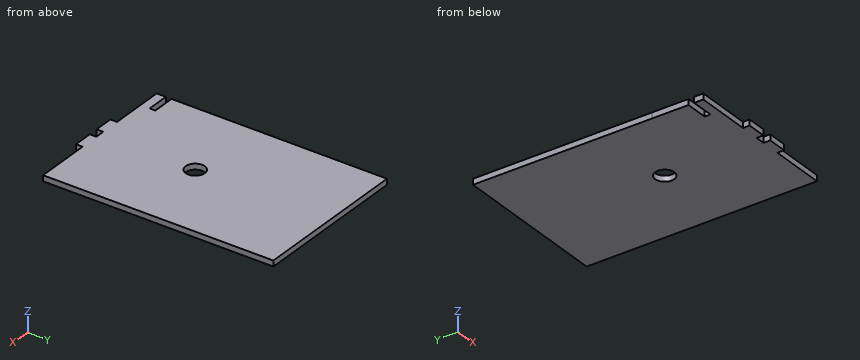
```python
from build123d import *

# Parameters (mm, degrees)
MODEL_R                 = 5
SALIENTE_EXTRUIR1_DEPTH = 3


with BuildPart() as part:
    # Model → Saliente-Extruir1 (new body)
    with BuildSketch(Plane.XY):
        Polygon((43.835480064, -35.842547763), (43.835480064, -32.349014415), (14.885477826, -32.340639111), (14.885479202, -27.550194175), (26.685480393, -27.550194175), (26.685480393, -24.550194175), (14.885480064, -24.550193732), (14.885483847, -5.553308235), (14.885503897, 88.349821578), (97.885505249, 88.349799035), (97.885505249, -32.347086905), (68.935480064, -32.349014415), (68.935480064, -35.842547763), (58.885480064, -35.842547763), (58.885480064, -32.342547763), (53.885480064, -32.342547763), (53.885480064, -35.842547763), align=None)
        with Locations((56.385505249, 17.649799035)):
            Circle(MODEL_R, mode=Mode.SUBTRACT)
    extrude(amount=SALIENTE_EXTRUIR1_DEPTH)


solid = part.part
```
The listing builds one solid part. Answer for the finished solid, in the listing's coordinates (mm). Give positions to 0.01 mm unless a question says otherwise; leave off trailing zeros. Order: outer loops, then holes, each group sorted by start corner. A loop starts at its lowest first (then second) coordinate and runs counter-clockwise, first axis right, second up. Notation, with made-up numbers: (-4.75, 36.25) - (9.25, 36.25) arc R19 cw to (9.25, 50.25) - close; hole circle Ø8 at (8.5, -26.5). An arc over 180 degrees is marked (long way). Use one line per item in the form item = value. Start each with the question number.
(1) A cutting plane is placed at A-A, the plane x = 57. Write down the section's boundary in (y, z).
(2) A cutting plane is placed at B-B, the plane z = 1.45. Write down the section's boundary in (x, y).
(3) Consider line 1 (Y direction, x = 91, z = 2.6); line 2 (X direction, y = -27, z = 2.3); line 3 (Y direction, x = 55, z = 1.3). Determine where each line is inside the solid, lowest interval first. Write a range as from..to.
(4) A cutting plane is placed at D-D, the plane x = 42. Write down the section's boundary in (y, z).
(5) A cutting plane is placed at C-C, the plane x = 29. Write down the section's boundary in (y, z).
(6) Flat-ended cylindrical pins translate along their axes: pin 1 Ø0.9 at (x, z) = (22.5, 2) entering from -Y; pin 2 Ø1.5 at (y, z) = (-34.5, 1.5) entering from +X; pin 3 Ø1.5 at (y, z) = (-33.5, 1) entering from -X; pin 4 Ø8 at (x, y) = (56.39, 17.65) entering from +Z. Find the tip coordinate at first contact, or state that the pin passes through.
Ans:
q1.outline = (-32.34, 0) - (12.69, 0) - (12.69, 3) - (-32.34, 3) - close; (22.61, 0) - (88.35, 0) - (88.35, 3) - (22.61, 3) - close
q2.outline = (14.89, -32.34) - (43.84, -32.35) - (43.84, -35.84) - (53.89, -35.84) - (53.89, -32.34) - (58.89, -32.34) - (58.89, -35.84) - (68.94, -35.84) - (68.94, -32.35) - (97.89, -32.35) - (97.89, 88.35) - (14.89, 88.35) - (14.89, -24.55) - (26.69, -24.55) - (26.69, -27.55) - (14.89, -27.55) - close; hole circle Ø10 at (56.39, 17.65)
q3.line_1 = -32.35..88.35
q3.line_2 = 26.69..97.89
q3.line_3 = -32.34..12.85, 22.45..88.35
q4.outline = (-32.35, 0) - (88.35, 0) - (88.35, 3) - (-32.35, 3) - close
q5.outline = (-32.34, 0) - (88.35, 0) - (88.35, 3) - (-32.34, 3) - close
q6.pin_1 = -32.34
q6.pin_2 = 68.94
q6.pin_3 = 43.84
q6.pin_4 = through
